Can you work these out from the model? Positions are in its coordinate system, mm. Face numbers are marked on the shaded views. A direction names the side the tool comes from. Coordinates: 2 decimals unless noted, no trailing zeros. Order: outer loops, then holes, each group sorted by start corner. A loop starts at its lowest first (then second) coordinate and runs counter-clockwise, first axis right, second up. Notation, with made-up numbers: (-17, 2.5) -> (39, 2.5) arc R5 cw to (39, 9.5) -> close; hole circle Ø2 at (71.5, 6.5). An arc over 180 degrees is marked (long way). Answer in a Markdown table with one row per item. Add a question column.
1. Imagine slicing it at C-C on y = 152. Write out the boundary of the cut face in (x, z).
2. Imagine slicing it at A-A on x = 22.5. Write out the boundary of the cut face in (y, z).
3. Imagine slicing it at D-D on x = 51. Write out the boundary of the cut face in (y, z).
4. We'd pull the mould along Y, two halves only. Please class the marked faces 4, 5 and 6: pulls with the +Y half, pulls with the -Y half, needs draft (parallel to the pull), parting line crosses it, or undercut.
5. Will these pins go through, and if not, where does the flat tip stop? pin 1 (6.5 mm diameter, centred on x = 50.5, z = -6.5, fed in from +Y); pin 2 (4 mm diameter, centred on y = 145.5, z = -5, fed in from +X); pin 3 (1.5 mm diameter, centred on y = 75.5, z = -10.5, fed in from -X).
6. If I drill on line 1 along Y through (x, z) = (9, -1.25); line 2 along Y through (x, z) = (42, -10.25); line 3 along X through (y, z) = (110, -12), over which ranges is the centre line in solid material (lowest first)? Write a range as [from, to].
7. On a 3-axis mill with a long thin cutter (end or side, diameter ignored), from which of +Z, -Z, +X, -X, +Y, -Y can I reach the whole of each face in a straight line? I mean the marked faces 1, 2 and 3. Say none if no direction works.
8. Imagine slicing it at B-B on z = -1.5. Write out the boundary of the cut face in (x, y).
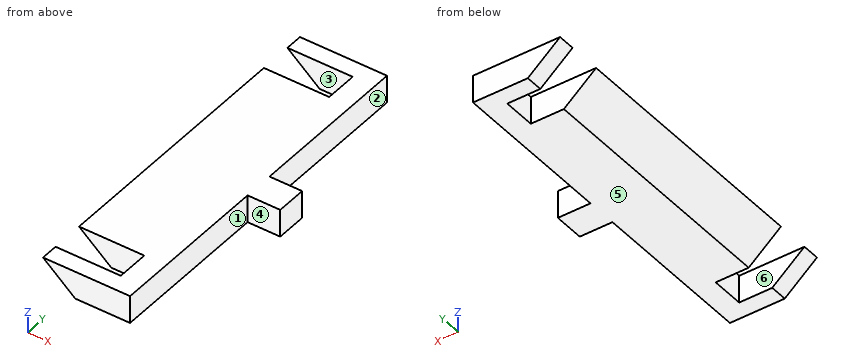
from build123d import *

# Parameters (mm, degrees)
SALIENTE_EXTRUIR1_DEPTH    = 170
CROQUIS2_W                 = 8
CROQUIS2_H                 = 27
CORTAR_EXTRUIR1_DEPTH      = 1
CORTAR_EXTRUIR1_DEPTH_BACK = 16
CROQUIS3_W                 = 38.06511858
CROQUIS3_H                 = 175.826127046
CORTAR_EXTRUIR2_DEPTH      = 1
CORTAR_EXTRUIR2_DEPTH_BACK = 16
CROQUIS4_W                 = 35.532251822
CROQUIS4_H                 = 7.536766594
CORTAR_EXTRUIR3_DEPTH      = 1
CORTAR_EXTRUIR3_DEPTH_BACK = 171
CROQUIS5_W                 = 14.817344245
CROQUIS5_H                 = 15
CROQUIS5_W_2               = 15.182655755
CROQUIS5_W_3               = 6
CROQUIS5_H_2               = 75
CROQUIS5_H_3               = 6
CORTAR_EXTRUIR4_DEPTH      = 1
CORTAR_EXTRUIR4_DEPTH_BACK = 13.7
CROQUIS6_W                 = 9
CROQUIS6_H                 = 14
SALIENTE_EXTRUIR2_DEPTH    = 12.7


with BuildPart() as part:
    # Croquis1 → Saliente-Extruir1 (new body)
    with BuildSketch(Plane(origin=(0, 0, 0), x_dir=(1, 0, 0), z_dir=(0, 1, 0))):
        Polygon((0, 0), (17.50080029, 15), (60, 15), (60, 0), align=None)
    extrude(amount=SALIENTE_EXTRUIR1_DEPTH)

    # Croquis2 → Cortar-Extruir1 (cut, two sides)
    with BuildSketch(Plane(origin=(0, 0, -15), x_dir=(-1, 0, 0), z_dir=(0, 0, -1))) as cortar_extruir1_sk:
        with Locations((-56, 13.5)):
            Rectangle(CROQUIS2_W, CROQUIS2_H)
        with Locations((-56, 156.5)):
            Rectangle(CROQUIS2_W, CROQUIS2_H)
    extrude(amount=CORTAR_EXTRUIR1_DEPTH, mode=Mode.SUBTRACT)
    extrude(cortar_extruir1_sk.sketch, amount=-CORTAR_EXTRUIR1_DEPTH_BACK, mode=Mode.SUBTRACT)

    # Croquis3 → Cortar-Extruir2 (cut, two sides)
    with BuildSketch(Plane(origin=(0, 0, -15), x_dir=(-1, 0, 0), z_dir=(0, 0, -1))) as cortar_extruir2_sk:
        with Locations((-65.03255929, 82.086936477)):
            Rectangle(CROQUIS3_W, CROQUIS3_H)
    extrude(amount=CORTAR_EXTRUIR2_DEPTH, mode=Mode.SUBTRACT)
    extrude(cortar_extruir2_sk.sketch, amount=-CORTAR_EXTRUIR2_DEPTH_BACK, mode=Mode.SUBTRACT)

    # Croquis4 → Cortar-Extruir3 (cut, two sides)
    with BuildSketch(Plane.XZ) as cortar_extruir3_sk:
        with Locations((28.233874089, -16.468383297)):
            Rectangle(CROQUIS4_W, CROQUIS4_H)
    extrude(amount=CORTAR_EXTRUIR3_DEPTH, mode=Mode.SUBTRACT)
    extrude(cortar_extruir3_sk.sketch, amount=-CORTAR_EXTRUIR3_DEPTH_BACK, mode=Mode.SUBTRACT)

    # Croquis5 → Cortar-Extruir4 (cut, two sides)
    with BuildSketch(Plane(origin=(0, 0, -12.7), x_dir=(-1, 0, 0), z_dir=(0, 0, -1))) as cortar_extruir4_sk:
        with Locations((-7.408672123, 21.5)):
            Rectangle(CROQUIS5_W, CROQUIS5_H)
        with Locations((-22.408672123, 21.5)):
            Rectangle(CROQUIS5_W_2, CROQUIS5_H)
        with Locations((-43, 43.5)):
            Rectangle(CROQUIS5_W_3, CROQUIS5_H_2)
        Polygon((-40, 6), (-46, 6), (-46, 0), (-14.817344245, 0), (-14.817344245, 6), align=None)
        with Locations((-7.408672123, 3)):
            Rectangle(CROQUIS5_W, CROQUIS5_H_3)
        with Locations((-43, 132.5)):
            Rectangle(CROQUIS5_W_3, CROQUIS5_H_2)
        with Locations((-22.408672123, 154.5)):
            Rectangle(CROQUIS5_W_2, CROQUIS5_H)
        with Locations((-7.408672123, 154.5)):
            Rectangle(CROQUIS5_W, CROQUIS5_H)
    extrude(amount=CORTAR_EXTRUIR4_DEPTH, mode=Mode.SUBTRACT)
    extrude(cortar_extruir4_sk.sketch, amount=-CORTAR_EXTRUIR4_DEPTH_BACK, mode=Mode.SUBTRACT)

    # Croquis6 → Saliente-Extruir2 (add)
    with BuildSketch(Plane(origin=(0, 0, -12.7), x_dir=(-1, 0, 0), z_dir=(0, 0, -1))):
        with Locations((-50.5, 88)):
            Rectangle(CROQUIS6_W, CROQUIS6_H)
    extrude(amount=-SALIENTE_EXTRUIR2_DEPTH)


solid = part.part
Answers follow:
| question | item | result |
|---|---|---|
| 1 | outline | (30, -12.7) -> (40, -12.7) -> (40, 0) -> (30, 0) -> close |
| 2 | outline | (6, -12.7) -> (14, -12.7) -> (14, 0) -> (6, 0) -> close; (29, -12.7) -> (147, -12.7) -> (147, 0) -> (29, 0) -> close; (162, -12.7) -> (170, -12.7) -> (170, 0) -> (162, 0) -> close |
| 3 | outline | (81, -12.7) -> (95, -12.7) -> (95, 0) -> (81, 0) -> close |
| 4 | face 4 | pulls with the -Y half |
| 4 | face 5 | needs draft |
| 4 | face 6 | undercut |
| 5 | pin 1 | stops at y = 95 |
| 5 | pin 2 | stops at x = 40 |
| 5 | pin 3 | stops at x = 11.38 |
| 6 | line 1 | y = [6, 14], [29, 147], [162, 170] |
| 6 | line 2 | y = [81, 95] |
| 6 | line 3 | x = [14, 40] |
| 7 | face 1 | +Z, -Z, +X, -Y |
| 7 | face 2 | +Z, -Z, +X, +Y |
| 7 | face 3 | +Z, -Z, -X |
| 8 | outline | (1.75, 6) -> (40, 6) -> (40, 81) -> (55, 81) -> (55, 95) -> (40, 95) -> (40, 170) -> (1.75, 170) -> (1.75, 162) -> (30, 162) -> (30, 147) -> (1.75, 147) -> (1.75, 29) -> (30, 29) -> (30, 14) -> (1.75, 14) -> close |
